The figure shows three views and two pictorial views of one solid part (mm, origin at its lowest corner). Answer the questions. A direction names the side the tool comes from. Coordinates: 2 decimals unless noted, no trailing zeros. Loops run counter-clockwise (first coordinate to the right, second up) from the corner with the lowest first, then second, coordinate; pieces in that order, holes last. Notation, with made-up numbers: M -15.75,-19.5 L 12.25,-19.5 A17 cw 12.25,0.5 Z; hole C -4,82.5 d9. An arc over 180 degrees is marked long. Answer in a Markdown table with one row per item. Add a question column.
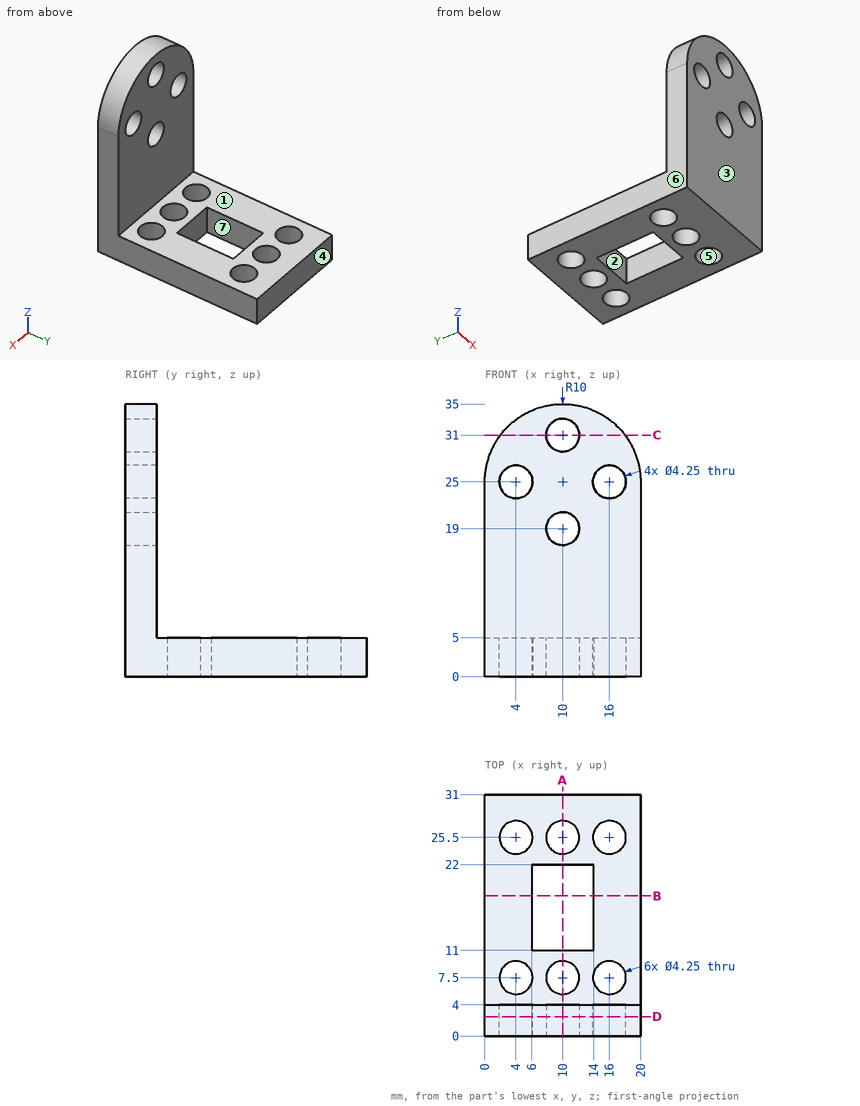
(1) Each of these flat-tipped pins is pushed along its axis until it touches: pin 1 (10 mm diameter, centred on x = 16.5, z = 13, fed in from +Y); pin 2 (4 mm diameter, centred on x = 16.5, y = 12, fed in from +Z); pin 3 (12 mm diameter, centred on y = 20.5, z = 9.5, fed in from +X). Where does it stop, or does it pass through?
(2) A cutting plane is placed at D-D (y = 2.5). Give the vertices of the cut face in (x, z) (3 decimals), plus the area to 3 significant figures.
(3) A cutting plane is placed at A-A (x = 10). Give the vertices of the cut face in (y, z) (3 decimals).
(4) A cutting plane is placed at B-B (y = 18). Give the vertices of the cut face in (x, z), plus the area to 3 significant figures.
(5) A cutting plane is placed at C-C (z = 31). Give the vertices of the cut face in (x, y) (3 decimals), plus the area to 3 significant figures.
(6) Straight lines are drawn through the part: line 1 (X direction, y = 25.5, z = 2.35) (3 decimals); line 2 (Y direction, x = 4, z = 1.1) (3 decimals); line 3 (Z direction, x = 10, y = 3.15) (3 decimals). For each, find the intervals that lie inside material, in ascending order.
(7) For the marked faces 1, 2 and 3, determine the directions among +Z, -Z, +X, -X, +Y, -Y from which every point of the face is accessible in a straight line to the end or side of a thin tool.
(8) The mould has two halves that part along X. Classify the marked faces 4, 5, 6 and 7: released by +X, released by -X, zero draft, split by the parting line, or undercut.
Solved:
| question | item | result |
|---|---|---|
| 1 | pin 1 | stops at y = 4 |
| 1 | pin 2 | stops at z = 5 |
| 1 | pin 3 | stops at x = 20 |
| 2 | outline | M 0,0 L 20,0 L 20,25 A10 ccw 0,25 Z; hole C 4,25 d4.25; hole C 10,19 d4.25; hole C 10,31 d4.25; hole C 16,25 d4.25 |
| 2 | area | 600 mm² |
| 3 | outline | M 0,0 L 5.375,0 L 5.375,5 L 4,5 L 4,16.875 L 0,16.875 Z; M 0,21.125 L 4,21.125 L 4,28.875 L 0,28.875 Z; M 0,33.125 L 4,33.125 L 4,35 L 0,35 Z; M 9.625,0 L 11,0 L 11,5 L 9.625,5 Z; M 22,0 L 23.375,0 L 23.375,5 L 22,5 Z; M 27.625,0 L 31,0 L 31,5 L 27.625,5 Z |
| 4 | outline | M 0,0 L 6,0 L 6,5 L 0,5 Z; M 14,0 L 20,0 L 20,5 L 14,5 Z |
| 4 | area | 60.0 mm² |
| 5 | outline | M 2,0 L 7.875,0 L 7.875,4 L 2,4 Z; M 12.125,0 L 18,0 L 18,4 L 12.125,4 Z |
| 5 | area | 47.0 mm² |
| 6 | line 1 | x = 0 to 1.875, 6.125 to 7.875, 12.125 to 13.875, 18.125 to 20 |
| 6 | line 2 | y = 0 to 5.375, 9.625 to 23.375, 27.625 to 31 |
| 6 | line 3 | z = 0 to 16.875, 21.125 to 28.875, 33.125 to 35 |
| 7 | face 1 | +Z, +X, -X, +Y |
| 7 | face 2 | +Z, -Z |
| 7 | face 3 | +Z, -Z, +X, -X, -Y |
| 8 | face 4 | zero draft |
| 8 | face 5 | undercut |
| 8 | face 6 | released by -X |
| 8 | face 7 | undercut |
